```python
from build123d import *

# Parameters (mm, degrees)
BOSS_EXTRUDE1_DEPTH = 10.8
BOSS_EXTRUDE2_DEPTH = 1
BOSS_EXTRUDE3_DEPTH = 0.9
SKETCH5_W           = 2
SKETCH5_H           = 2.5
CUT_EXTRUDE1_DEPTH  = 5.2
CUT_EXTRUDE2_DEPTH  = 3.75
SKETCH7_W           = 1
SKETCH7_H           = 1
CUT_EXTRUDE3_DEPTH  = 2.5
FILLET1_R           = 0.1
CHAMFER1_SIZE       = 0.1


with BuildPart() as part:
    # Sketch2 → Boss-Extrude1 (new body)
    with BuildSketch(Plane(origin=(0, 0, 0), x_dir=(0, 0, -1), z_dir=(1, 0, 0))):
        Polygon((0, 4.116746825), (6.25, 4.116746825), (6.53, 3.836746825), (6.53, 2.066746825), (6.56, 2.066746825), (6.84, 1.786746825), (6.84, 0), (0, 0), align=None)
    extrude(amount=BOSS_EXTRUDE1_DEPTH)

    # Sketch3 → Boss-Extrude2 (add)
    with BuildSketch(Plane.XY):
        Polygon((-0.9, 1.016746825), (-0.9, -0.883253175), (11.7, -0.883253175), (11.7, 4.116746825), (-0.9, 4.116746825), (-0.9, 2.216746825), (-0.3, 1.616746825), align=None)
    extrude(amount=BOSS_EXTRUDE2_DEPTH)

    # Sketch4 → Boss-Extrude3 (add)
    with BuildSketch(Plane(origin=(0, 4.116746825, 0), x_dir=(1, 0, 0), z_dir=(0, 1, 0))):
        Polygon((1.249253009, 2.891399382), (0.893756458, 3.03935436), (0.893756458, 3.77625502), (1.41465396, 4.678475961), (1.993020778, 4.678475961), (1.993020778, -0.09), (8.806979222, -0.09), (8.806979222, 4.678475961), (9.38534604, 4.678475961), (9.906243542, 3.77625502), (9.906243542, 3.03935436), (9.550746991, 2.891399382), (9.045115198, -1), (1.754884802, -1), align=None)
    extrude(amount=BOSS_EXTRUDE3_DEPTH)

    # Sketch5 → Cut-Extrude1 (cut)
    with BuildSketch(Plane.XY.offset(1)):
        with Locations((1.65, 2.066746825)):
            Rectangle(SKETCH5_W, SKETCH5_H)
        with Locations((4.15, 2.066746825)):
            Rectangle(SKETCH5_W, SKETCH5_H)
        with Locations((6.65, 2.066746825)):
            Rectangle(SKETCH5_W, SKETCH5_H)
        with Locations((9.15, 2.066746825)):
            Rectangle(SKETCH5_W, SKETCH5_H)
    extrude(amount=-CUT_EXTRUDE1_DEPTH, mode=Mode.SUBTRACT)

    # Sketch6 → Cut-Extrude2 (cut)
    with BuildSketch(Plane(origin=(0, 0, -6.84), x_dir=(-1, 0, 0), z_dir=(0, 0, -1))):
        Polygon((-9.55, 0.8), (-8.75, 0.8), (-8.55, 0), (-9.75, 0), align=None)
        Polygon((-7.05, 0.8), (-6.25, 0.8), (-6.05, 0), (-7.25, 0), align=None)
        Polygon((-4.55, 0.8), (-3.75, 0.8), (-3.55, 0), (-4.75, 0), align=None)
        Polygon((-2.05, 0.8), (-1.25, 0.8), (-1.05, 0), (-2.25, 0), align=None)
    extrude(amount=-CUT_EXTRUDE2_DEPTH, mode=Mode.SUBTRACT)

    # Sketch7 → Cut-Extrude3 (cut)
    with BuildSketch(Plane(origin=(0, 0, -6.53), x_dir=(-1, 0, 0), z_dir=(0, 0, -1))):
        with Locations((-9.15, 2.836746825)):
            Rectangle(SKETCH7_W, SKETCH7_H)
        with Locations((-6.65, 2.836746825)):
            Rectangle(SKETCH7_W, SKETCH7_H)
        with Locations((-4.15, 2.836746825)):
            Rectangle(SKETCH7_W, SKETCH7_H)
        with Locations((-1.65, 2.836746825)):
            Rectangle(SKETCH7_W, SKETCH7_H)
    extrude(amount=-CUT_EXTRUDE3_DEPTH, mode=Mode.SUBTRACT)

    # Fillet1
    fillet1_edges = [part.edges().sort_by_distance(p)[0] for p in [
        (9.297931094, 5.016746825, -0.945699691),
        (9.728495267, 5.016746825, -2.965376871),
        (9.906243542, 5.016746825, -3.40780469),
        (9.645794791, 5.016746825, -4.22736549),
        (9.096162631, 5.016746825, -4.678475961),
        (8.806979222, 5.016746825, -2.29423798),
        (5.4, 5.016746825, 0.09),
        (1.993020778, 5.016746825, -2.29423798),
        (1.703837369, 5.016746825, -4.678475961),
        (1.154205209, 5.016746825, -4.22736549),
        (0.893756458, 5.016746825, -3.40780469),
        (1.071504733, 5.016746825, -2.965376871),
        (1.502068906, 5.016746825, -0.945699691),
        (-0.6, 1.916746825, 0),
        (-0.6, 1.316746825, 1),
        (0, 0, -3.42),
        (0, 4.116746825, -3.125),
        (10.8, 0, -3.42),
        (-0.45, 4.116746825, 0),
        (-0.9, 3.166746825, 0),
        (-0.6, 1.316746825, 0),
        (-0.9, 0.066746825, 0),
        (5.4, -0.883253175, 0),
        (11.25, 4.116746825, 0),
        (11.7, 1.616746825, 0),
        (10.372557599, 4.116746825, 1),
        (-0.9, 0.066746825, 1),
        (-0.6, 1.916746825, 1),
        (-0.9, 3.166746825, 1),
        (0.427442401, 4.116746825, 1),
        (5.4, -0.883253175, 1),
        (11.7, 1.616746825, 1),
        (-0.3, 1.616746825, 0.5),
        (-0.9, 1.016746825, 0.5),
        (-0.9, 2.216746825, 0.5),
        (-0.9, 4.116746825, 0.5),
        (-0.9, -0.883253175, 0.5),
        (11.7, -0.883253175, 0.5),
        (10.8, 4.116746825, -3.125),
        (11.7, 4.116746825, 0.5),
        (0.525, 0, -6.84),
        (2.9, 0, -6.84),
        (5.4, 0, -6.84),
        (7.9, 0, -6.84),
        (10.275, 0, -6.84),
    ]]
    fillet(fillet1_edges, radius=FILLET1_R)

    # Chamfer1
    chamfer1_edges = [part.edges().sort_by_distance(p)[0] for p in [
        (3.15, 2.066746825, 1),
        (4.15, 0.816746825, 1),
        (5.15, 2.066746825, 1),
        (4.15, 3.316746825, 1),
        (5.65, 2.066746825, 1),
        (6.65, 0.816746825, 1),
        (7.65, 2.066746825, 1),
        (6.65, 3.316746825, 1),
        (8.15, 2.066746825, 1),
        (9.15, 0.816746825, 1),
        (10.15, 2.066746825, 1),
        (9.15, 3.316746825, 1),
        (9.65, 2.836746825, -6.53),
        (9.15, 2.336746825, -6.53),
        (8.65, 2.836746825, -6.53),
        (9.15, 3.336746825, -6.53),
        (7.15, 2.836746825, -6.53),
        (6.65, 2.336746825, -6.53),
        (6.15, 2.836746825, -6.53),
        (6.65, 3.336746825, -6.53),
        (4.65, 2.836746825, -6.53),
        (4.15, 2.336746825, -6.53),
        (3.65, 2.836746825, -6.53),
        (4.15, 3.336746825, -6.53),
        (2.15, 2.836746825, -6.53),
        (1.65, 2.336746825, -6.53),
        (1.15, 2.836746825, -6.53),
        (1.65, 3.336746825, -6.53),
        (0.65, 2.066746825, 1),
        (1.65, 0.816746825, 1),
        (2.65, 2.066746825, 1),
        (1.65, 3.316746825, 1),
    ]]
    chamfer(chamfer1_edges, length=CHAMFER1_SIZE)


solid = part.part
```
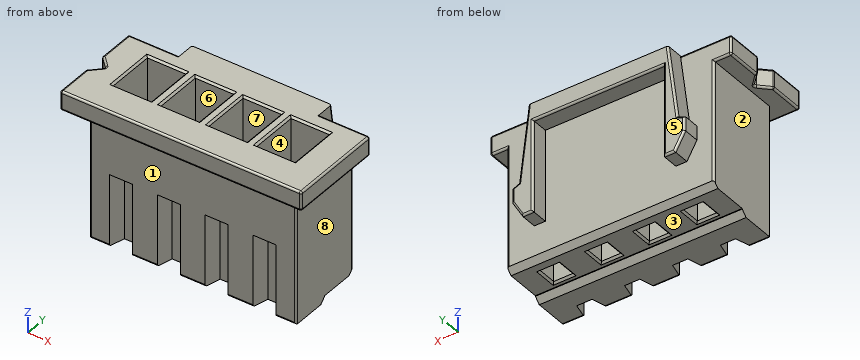
Geometry: final body of the model. Coordinates: model frame, mm. Face numbers are marked on the shaded views. A direction names the side the tool comes from. Round coordinates to 2 decimals unless told otherwise and drop trailing zeros. Write each loop counter-clockwise with the first axis right and the second up, starting at its lowest first coordinate (ties: lowest second). Pieces come first, ordered by that corner, then holes. Notation, with made-up numbers: (62.5, 24.25) -> (76.5, 24.25) arc R23 cw to (76.5, 44.25) -> close; hole circle Ø8 at (66, -8.75). An arc over 180 degrees is marked (long way). Use CSV: the item, a comma, the result in double quotes. Start each with the question number.
Q1. Reachability of the marked faces 1, 2, 3 and 4 from +Z, -Z, +X, -X, +Y, -Y: full face, straight path, thin tool, end or side. Return the list, or none.
Q2. Pull-direction query (Y, two-part tool) for the marked faces 5, 6, 7 and 8; classes: pulls with the +Y half, pulls with the -Y half, needs draft (parallel to the pull), parting line crosses it, or undercut.
Q3. Section C-C (z = -5.25). Give the number of separate pieces and of enclosed holes in the cut face, plus the area to 3 significant figures.
Q4. Section D-D (y = -0.45). Return loops of the section in (x, z), plus the area to 3 significant figures.
Q5. First-contact query: pin 1 Ø0.6 at (x, z) = (6.5, -0.5) entering from -Y; pin 2 Ø1.2 at (y, z) = (2, -1.5) entering from -X; pin 3 Ø4 at (x, z) = (7, -4) entering from +Y; pin 4 Ø0.8 at (y, z) = (2.5, -4.5) entering from +X. Flat tips, straight axial feed; report the tip coordinate or a pass-through.
Q6. Section B-B (y = 4.3). Return loops of the section in (x, z), plus the area to 3 significant figures.
Q7. Line query: L1, parallel to X at y = 2.6, z = -4.5; L2, parallel to X at y = 2.2, z = 0.5; L3, parallel to Y at x = 1.5, z = -5. Output: solid intervals per line, ascending.
Result sheet:
1,face 1,"-Z, +X, -X, -Y"
1,face 2,"-Z, -X, +Y, -Y"
1,face 3,"-Z, +X, -X, +Y"
1,face 4,"+Z"
2,face 5,"pulls with the +Y half"
2,face 6,"undercut"
2,face 7,"undercut"
2,face 8,"needs draft"
3,separate pieces,"1"
3,enclosed holes,"4"
3,area,"37.3 mm²"
4,outline,"(-0.9, 0.1) arc R0.1 ccw to (-0.8, 0) -> (11.6, 0) arc R0.1 ccw to (11.7, 0.1) -> (11.7, 0.9) arc R0.1 ccw to (11.6, 1) -> (-0.8, 1) arc R0.1 ccw to (-0.9, 0.9) -> close"
4,area,"12.6 mm²"
5,pin 1,"y = 0"
5,pin 2,"x = 0"
5,pin 3,"y = 5.02"
5,pin 4,"x = 10.8"
6,outline,"(0.89, -3.78) -> (1.41, -4.68) -> (1.99, -4.68) -> (1.99, 0.09) -> (8.81, 0.09) -> (8.81, -4.68) -> (9.39, -4.68) -> (9.91, -3.78) -> (9.91, -3.04) -> (9.55, -2.89) -> (9.05, 1) -> (1.75, 1) -> (1.25, -2.89) -> (0.89, -3.04) -> close"
6,area,"13.4 mm²"
7,L1,"0 to 1.15, 2.15 to 3.65, 4.65 to 6.15, 7.15 to 8.65, 9.65 to 10.8"
7,L2,"-0.88 to 0.65, 2.65 to 3.15, 5.15 to 5.65, 7.65 to 8.15, 10.15 to 11.7"
7,L3,"0.8 to 2.34, 3.34 to 4.12"
